Verification items for the finished model (mm, model axes). A direction names the side the tool comes from. Give positions to 0.01 mm unless a question says otherwise; leave off trailing zeros. Loops run counter-clockwise (first coordinate to the right, second up) from the corner with the lowest first, then second, coordinate; pieces in that order, holes last. Notation, with made-up numbers: (38, -28) - (49, -28) arc R33 ccw to (49, 1) - close; hole circle Ø3 at (-31, 18). An arc over 180 degrees is marked (long way). Use one line per item in the form item = value.
```python
from build123d import *

# Parameters (mm, degrees)
P_IDAT_VYSUNUT_M1_DEPTH       = 3.6
ODEBRAT_VYSUNUT_M1_DEPTH      = 3
ODEBRAT_VYSUNUT_M1_DEPTH_BACK = 4
P_IDAT_VYSUNUT_M2_DEPTH       = 2.5
LINPOLE1_COUNT                = 12
LINPOLE1_PITCH                = 1.9
LINPOLE1_COL_COUNT            = 3
LINPOLE1_COL_PITCH            = 1.9
SKICA5_R                      = 0.95
ODEBRAT_VYSUNUT_M2_DEPTH      = 5


with BuildPart() as part:
    # Skica1 → Přidat vysunutím1 (new body)
    with BuildSketch(Plane.XY):
        Polygon((0, 0), (0, -3), (8, -3), (8.595876796, -2.5), (35, -2.5), (37.598076211, 2), (35.598076211, 2), (33.598076211, 0), align=None)
    extrude(amount=P_IDAT_VYSUNUT_M1_DEPTH)

    # Skica2 → Odebrat vysunutím1 (cut, two sides)
    with BuildSketch(Plane(origin=(0, 0, 0), x_dir=(1, 0, 0), z_dir=(0, 1, 0))) as odebrat_vysunut_m1_sk:
        Polygon((8, 0), (8.595876796, -0.4), (37.598076211, -0.4), (37.598076211, 0), align=None)
    extrude(amount=ODEBRAT_VYSUNUT_M1_DEPTH, mode=Mode.SUBTRACT)
    extrude(odebrat_vysunut_m1_sk.sketch, amount=-ODEBRAT_VYSUNUT_M1_DEPTH_BACK, mode=Mode.SUBTRACT)

    # Skica3 → Přidat vysunutím2 (add)
    with BuildSketch(Plane(origin=(0, -4.2, 3.6), x_dir=(1, 0, 0), z_dir=(0, 0, -1))):
        Polygon((9.295876796, -4.2), (10.195876796, -4.2), (9.995876796, -5.7), (9.495876796, -5.7), align=None)
    p_idat_vysunut_m2 = extrude(amount=P_IDAT_VYSUNUT_M2_DEPTH)

    # LinPole1: Přidat vysunutím2 ×12
    with Locations(*[(i * LINPOLE1_PITCH, 0, 0) for i in range(1, LINPOLE1_COUNT)]):
        add(p_idat_vysunut_m2)

    # LinPole1 col: Přidat vysunutím2 ×3
    with Locations(*[(-i * LINPOLE1_COL_PITCH, 0, 0) for i in range(1, LINPOLE1_COL_COUNT)]):
        add(p_idat_vysunut_m2)

    # Skica5 → Odebrat vysunutím2 (cut)
    with BuildSketch(Plane.XZ.offset(3)):
        with Locations((3.314552363, 2.006068977)):
            Circle(SKICA5_R)
    extrude(amount=-ODEBRAT_VYSUNUT_M2_DEPTH, mode=Mode.SUBTRACT)


solid = part.part
```
1. Scan lines: probe 1 along Z at (x, y) = (31, -1.95); probe 2 along Y at (x, z) = (7.5, 0.85); probe 3 along Y at (x, z) = (27, 1.4). Record each from-to range of solid material in increasing order.
Result set:
probe_1 = 0.4 to 3.6
probe_2 = -3 to 0
probe_3 = -2.5 to 1.5
2. Tool access check on faces 4 (the flat face through (17, 0, 0.6)), 5 (the flat face through (21, 1, 1.1)), 6 (the flat face through (7.497, 0.76, 2.368)). Record the directions out of +Z, -Z, +X, -X, +Y, -Y that give a thin tool (end or side, any length) a straight path to the whole face; none if there is none.
Result set:
face_4 = -Z, +Y
face_5 = -Z, -X, +Y
face_6 = +Z, -Z, +Y
3. Depth check by flat-ended pin: pin 1 Ø1.5 at (x, z) = (27, 1) entering from -Y; pin 2 Ø1.4 at (x, y) = (30, 0.5) entering from -Z; pin 3 Ø0.7 at (x, y) = (29, 0.5) entering from -Z. Enter the tip coordinate at first touch or a pass-through.
Result set:
pin_1 = -2.5
pin_2 = 0.4
pin_3 = 1.1
4. Draft check along X on faces 1 (the flat face through (19.3, 0.7, 1.1)), 2 (the flat face through (0, -1, 2)), 3 (the flat face through (17.697, 0.74, 2.368)). Enter one of: released by +X, released by -X, zero draft, split by the parting line, or undercut.
Result set:
face_1 = zero draft
face_2 = released by -X
face_3 = undercut
5. Section check C-C, the plane y = 0.6. State how many separate pieces and enclosed holes the cut face has, then the cut area to 3 significant figures.
Result set:
separate_pieces = 15
enclosed_holes = 0
area = 34.2 mm²
6. Section check A-A, the plane y = -2.05. Record the cut outline in (x, z), then the cut area to 3 significant figures.
Result set:
outline = (0, 0) - (8, 0) - (8.6, 0.4) - (35.26, 0.4) - (35.26, 3.6) - (0, 3.6) - close; hole circle Ø1.9 at (3.31, 2.01)
area = 113 mm²
7. Section check B-B, the plane x = 12.5. Record the cut outline in (y, z).
Result set:
outline = (-2.5, 0.4) - (0, 0.4) - (0, 3.6) - (-2.5, 3.6) - close
